```python
from build123d import *

# Parameters (mm, degrees)
SKETCH2_R           = 2.5
SKETCH2_R_2         = 2
BOSS_EXTRUDE2_DEPTH = 30
SKETCH4_R           = 23.491441723
BOSS_EXTRUDE4_DEPTH = 2


with BuildPart() as part:
    # Sketch1 → Revolve1 (revolve)
    with BuildSketch(Plane.XY, mode=Mode.PRIVATE) as revolve1_sk:
        with BuildLine():
            Line((3.119266055, -4.816513761), (13.119266055, -4.816513761))
            Line((13.119266055, -4.816513761), (13.119266055, -2.816513761))
            Line((13.119266055, -2.816513761), (3.257916771, -2.816513761))
            ThreePointArc((3.257916771, -2.816513761), (-4.025816821, -0.658797724), (-10.372175668, 3.516396035))
            ThreePointArc((-10.372175668, 3.516396035), (-13.131249362, 6.018603225), (-16.672681055, 7.172635302))
            ThreePointArc((-16.672681055, 7.172635302), (-17.771282031, 6.282087215), (-16.880733945, 5.183486239))
            ThreePointArc((-16.880733945, 5.183486239), (-14.048292509, 4.237555299), (-11.880733945, 2.183486239))
            ThreePointArc((-11.880733945, 2.183486239), (-4.911005239, -2.452809391), (3.119266055, -4.816513761))
        make_face()
    revolve(revolve1_sk.sketch.rotate(Axis((13.119266055, -2.816513761, 0), (0, -1, 0)), 270), axis=Axis((13.119266055, -2.816513761, 0), (0, -1, 0)))

    # Sketch2 → Boss-Extrude2 (add)
    # profile 1 of 3: a face of its own
    with BuildSketch(Plane(origin=(0, -2.816513761, 0), x_dir=(1, 0, 0), z_dir=(0, 1, 0))):
        with Locations(Location((9.455762685, 3.402755216, 0), (0, 0, 270))):
            Circle(SKETCH2_R)
        with Locations(Location((9.455762685, 3.402755216, 0), (0, 0, 270))):
            Circle(SKETCH2_R_2, mode=Mode.SUBTRACT)
    # profile 2 of 3: a face of its own
    with BuildSketch(Plane(origin=(0, -2.816513761, 0), x_dir=(1, 0, 0), z_dir=(0, 1, 0))):
        with Locations(Location((17.8978902, 1.471309377, 0), (0, 0, 270))):
            Circle(SKETCH2_R)
        with Locations(Location((17.8978902, 1.471309377, 0), (0, 0, 270))):
            Circle(SKETCH2_R_2, mode=Mode.SUBTRACT)
    # profile 3 of 3: a face of its own
    with BuildSketch(Plane(origin=(0, -2.816513761, 0), x_dir=(1, 0, 0), z_dir=(0, 1, 0))):
        with Locations(Location((12.00414528, -4.874064593, 0), (0, 0, 270))):
            Circle(SKETCH2_R)
        with Locations(Location((12.00414528, -4.874064593, 0), (0, 0, 270))):
            Circle(SKETCH2_R_2, mode=Mode.SUBTRACT)
    extrude(amount=BOSS_EXTRUDE2_DEPTH)

    # Sketch4 → Boss-Extrude4 (add)
    with BuildSketch(Plane(origin=(0, 2, 0), x_dir=(1, 0, 0), z_dir=(0, 1, 0))):
        with Locations(Location((13.119266055, 0, 0), (0, 0, 270))):
            Circle(SKETCH4_R)
    extrude(amount=BOSS_EXTRUDE4_DEPTH)


solid = part.part
```
Model file for the job. Use its own axes, mm. A direction names the side the tool comes from. Round coordinates to 2 decimals unless told otherwise and drop trailing zeros. Loops run counter-clockwise (first coordinate to the right, second up) from the corner with the lowest first, then second, coordinate; pieces in that order, holes last. Notation, with made-up numbers: M 65.5,-29 L 101.5,-29 A32 ccw 101.5,6 Z; hole C -9,0 d11. An arc over 180 degrees is marked long. Put each result on its own line as item: value. Start each with the question number.
Item 1: Mould opens along X. For faces 4 (the face through (13, -4.817, 0)), 5 (the face through (12, 4, 5)) say: released by +X, released by -X, zero draft, split by the parting line, or undercut.
Item 2: Drill centre lines: line 1 along X through (y, z) = (8, -2); line 2 along Y through (x, z) = (13.5, 23); line 3 along Y through (x, z) = (-8, 0.5). Where is each one in solid material? Low to high.
Item 3: Drop flat-ended pins along their axis: P1, Ø1.5, axis at y = 5, z = -23, coming from the -X side; P2, Ø1, axis at x = 3.5, y = 2.5, coming from the -Z side; P3, Ø4.5, axis at x = 12.5, z = 5.5, coming from the +Y side; P4, Ø2, axis at x = 17.5, z = -1, coming from the +Y side. Give the stop position or say it passes through.
Item 4: Cut at A-A (y = 16.5). List the corners of the cut face in (x, z), then the cut area to 3 significant figures.
Item 5: 3-axis set-ups, long thin cutter, end or side, ignore diameter. For faces 1 (the face through (12.605, -0.442, 6.782)), 2 (the face through (11, 27.183, -5)), 3 (the face through (9, 4, -3)): which of +Z, -Z, +X, -X, +Y, -Y reach the whole face in a straight line?
Item 6: Cut at B-B (z = 6). Give the number of separate pieces and of enclosed holes in the cut face, then the cut area to 3 significant figures.
Answer block:
1. face 4: zero draft
1. face 5: undercut
2. line 1: 7.39 to 8.03, 10.88 to 11.53, 15.45 to 15.97, 19.83 to 20.34
2. line 2: 0.53 to 4
2. line 3: -0.76 to 1.64, 2 to 4
3. P1: x = -7.74
3. P2: z = -23.81
3. P3: y = 27.18
3. P4: y = 4
4. outline: C 9.46,-3.4 d5; C 12,4.87 d5; C 17.9,-1.47 d5; hole C 9.46,-3.4 d4; hole C 12,4.87 d4; hole C 17.9,-1.47 d4
4. area: 21.2 mm2
5. face 1: none
5. face 2: +Z, -Z, +X, -X, +Y
5. face 3: +Y
6. separate pieces: 1
6. enclosed holes: 3
6. area: 253 mm2
